```python
from build123d import *

# Parameters (mm, degrees)
F0_W        = 100
F0_H        = 50
F1_DEPTH    = 25
F2_W        = 10
F2_H        = 50
F3_DEPTH    = 0.5
F4_W        = 100
F4_H        = 50
F5_DEPTH    = 10
F6_T        = 2.5
F6_T3_DEPTH = 55
F7_R        = 5
F8_W        = 5
F8_H        = 20
F9_DEPTH    = 4.5
F10_W       = 15
F10_H       = 30
F10_W_2     = 5
F10_H_2     = 20
F11_DEPTH   = 1
F13_DEPTH   = 10


# Not quite as in the source:
# - a shell that OpenCascade refuses in one call is made with other operations: the cavity is built on its own and cut out


with BuildPart() as f1:
    # F0 (on Top) → F1 (new body)
    with BuildSketch(Plane.XY):
        Rectangle(F0_W, F0_H)
    extrude(amount=F1_DEPTH)

    # F2 (on Top) → F3 (join)
    with BuildSketch(Plane.XY):
        with Locations((-55, 0)):
            Rectangle(F2_W, F2_H)
    extrude(amount=F3_DEPTH)

    # F4 (on Top) → F5 (join)
    with BuildSketch(Plane.XY):
        with Locations((-110, 0)):
            Rectangle(F4_W, F4_H)
    extrude(amount=F5_DEPTH)

    # F6: shell of thickness 2.5, made by hand


with BuildPart() as f6_core1:
    # F6_t2: copy of F1
    add(f1.part)

    # the walls: a layer under each face that stays
    f6_faces = [f6_core1.faces().sort_by_distance(p)[0] for p in [
        (-50, 0, 12.75),
        (15, 25, 20.8333333333),
        (-160, 0, 5),
        (-110, 0, 10),
        (-60, 0, 5.25),
        (50, 0, 12.5),
        (0, 0, 25),
        (-125, -25, 4.1666666667),
        (-55, 0, 0.5),
    ]]
    thicken(f6_faces, amount=-F6_T, mode=Mode.SUBTRACT)

    # F6_s4 → F6_t3 (cut)
    with BuildSketch(Plane.XZ.offset(-27.5)):
        Polygon((-50.025, 0.525), (-47.5, 0.5), (-47.5, -2), (-50, -2), align=None)
        Polygon((-59.975, 0.525), (-62.5, 0.5), (-62.5, -2), (-60, -2), align=None)
    extrude(amount=F6_T3_DEPTH, mode=Mode.SUBTRACT)


with BuildPart() as f1_1:
    add(f1.part)

    # what is left inside the walls is the cavity
    f6_cavity = [f6_core1.part.solids().sort_by_distance(p)[0] for p in [
        (0, -7.5, 22.475),
        (-110, -7.5, 7.475),
    ]]
    add(f6_cavity, mode=Mode.SUBTRACT)

    # F7
    f7_edges = [f1_1.edges().sort_by_distance(p)[0] for p in [
        (-157.5, -22.5, 3.75),
        (-62.5, -22.5, 3.75),
        (-62.5, 22.5, 3.75),
        (-157.5, 22.5, 3.75),
        (-47.5, -22.5, 11.25),
        (47.5, -22.5, 11.25),
        (47.5, 22.5, 11.25),
        (-47.5, 22.5, 11.25),
    ]]
    fillet(f7_edges, radius=F7_R)

    # F8 (on Top) → F9 (join)
    with BuildSketch(Plane.XY):
        with Locations((52.5, 0)):
            Rectangle(F8_W, F8_H)
    extrude(amount=F9_DEPTH)

    # F10 (on Top) → F11 (join)
    with BuildSketch(Plane.XY):
        with Locations((-167.5, 0)):
            Rectangle(F10_W, F10_H)
        with Locations((-167.5, 0)):
            Rectangle(F10_W_2, F10_H_2, mode=Mode.SUBTRACT)
    extrude(amount=F11_DEPTH)

    # F12 (on Front) → F13 (join, symmetric)
    with BuildSketch(Plane.XZ):
        Polygon((55, 4.5), (54.5669872981, 5.25), (54.1339745962, 4.5), align=None)
    extrude(amount=F13_DEPTH, both=True)


solid = f1_1.part
```
The model under review builds one solid part; all positions refer to its coordinate system, in mm. A direction names the side the tool comes from. Give positions to 0.01 mm unless a question says otherwise; leave off trailing zeros. Write each loop counter-clockwise with the first axis right and the second up, starting at its lowest first coordinate (ties: lowest second). Pieces come first, ordered by that corner, then holes. Notation, with made-up numbers: (45, 70) -> (86, 70) arc R38 cw to (86, 108) -> close; hole circle Ø5 at (55, 0). An arc over 180 degrees is marked (long way). Put each result on its own line as item: value.
(1) We need section A-A, the plane z = 12.25. Give the boundary of the cut face in (x, y).
Results are:
outline: (-50, -25) -> (50, -25) -> (50, 25) -> (-50, 25) -> close; hole (-47.5, -17.5) arc R5 ccw to (-42.5, -22.5) -> (42.5, -22.5) arc R5 ccw to (47.5, -17.5) -> (47.5, 17.5) arc R5 ccw to (42.5, 22.5) -> (-42.5, 22.5) arc R5 ccw to (-47.5, 17.5) -> close
(2) We need section C-C, the plane x = -128. Give the boundary of the cut face in (y, z), and give its area (4 significant figures).
Results are:
outline: (-25, 0) -> (-22.5, 0) -> (-22.5, 7.5) -> (22.5, 7.5) -> (22.5, 0) -> (25, 0) -> (25, 10) -> (-25, 10) -> close
area: 162.5 mm²
(3) Tool access review of faces 4 (the cylindrical face through (46, -21.07, 11.09)), 5 (the flat face through (-60, 0, 5)), 6 (the flat face through (52, 10, 3)): name each direction out of +Z, -Z, +X, -X, +Y, -Y from which nothing blocks a thin tool from reaching the whole face with its end or side.
Results are:
face 4: -Z
face 5: +Z, +Y, -Y
face 6: +Z, -Z, +X, +Y
(4) For pin 1 Ø7.5 at (x, y) = (-171, 4.5) entering from +Z; pin 2 Ø4 at (x, y) = (-46, 12.5) entering from -Z; pin 3 Ø5 at (x, y) = (-121.5, -16.5) entering from +Z; pin 4 Ø13.5 at (x, y) = (-98, 5.5) entering from -Z, all flat-tipped, find the tip position at first contact; note any pin that passes through.
Results are:
pin 1: z = 1
pin 2: z = 0
pin 3: z = 10
pin 4: z = 7.5
(5) We need section B-B, the plane y = 8. Give the boundary of the cut face in (x, z).
Results are:
outline: (-175, 0) -> (-170, 0) -> (-170, 1) -> (-175, 1) -> close; (-165, 0) -> (-157.5, 0) -> (-157.5, 7.5) -> (-62.5, 7.5) -> (-62.5, 0) -> (-47.5, 0) -> (-47.5, 22.5) -> (47.5, 22.5) -> (47.5, 0) -> (55, 0) -> (55, 4.5) -> (54.57, 5.25) -> (54.13, 4.5) -> (50, 4.5) -> (50, 25) -> (-50, 25) -> (-50, 0.5) -> (-60, 0.5) -> (-60, 10) -> (-160, 10) -> (-160, 1) -> (-165, 1) -> close
(6) The part is to be moulded in two halves that separate along X. For faces 1 (the flat face through (55, 0, 2)), 2 (the flat face through (52, -10, 3)), 3 (the flat face through (-111, 22.5, 4)), say which applies: pulls with the +X half, pulls with the -X half, needs draft (parallel to the pull), parting line crosses it, or undercut.
Results are:
face 1: pulls with the +X half
face 2: needs draft
face 3: undercut
(7) We need section D-D, the plane y = -20.5. Give the boundary of the cut face in (x, z).
Results are:
outline: (-160, 0) -> (-156.5, 0) -> (-156.5, 7.5) -> (-63.5, 7.5) -> (-63.5, 0) -> (-46.5, 0) -> (-46.5, 22.5) -> (46.5, 22.5) -> (46.5, 0) -> (50, 0) -> (50, 25) -> (-50, 25) -> (-50, 0.5) -> (-60, 0.5) -> (-60, 10) -> (-160, 10) -> close
(8) To check wall thickness, follow probe 1 along X at (y, z) = (4, 5.5); probe 2 along X at (y, z) = (-9, 4.25); probe 3 along Y at (x, z) = (-146, 2). State the ranges of each line that lie inside material, in increasing order. Write a range as from..to.
Results are:
probe 1: -160..-157.5, -62.5..-60, -50..-47.5, 47.5..50
probe 2: -160..-157.5, -62.5..-60, -50..-47.5, 47.5..55
probe 3: -25..-22.5, 22.5..25
